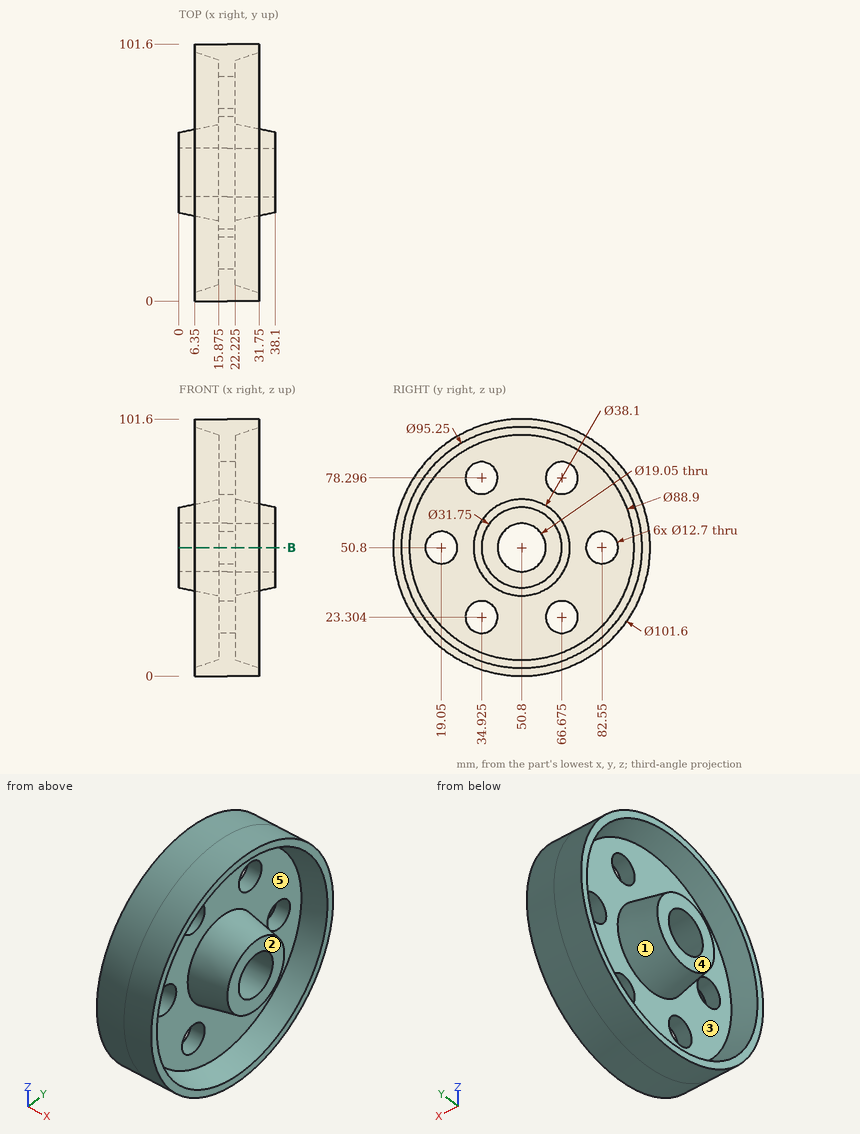
Answer from the drawing. Dimensions are ordinates in mm from the lowest x, y and z of the part. A direction names the side the tool comes from. Give positions to 0.01 mm unless a question says otherwise; leave off trailing zeros.
Item 1: Each of these flat-tipped pins is pushed along its axis until it touches: pin 1 Ø20.5 at (y, z) = (66.68, 23.3) entering from +X (3 decimals); pin 2 Ø1 at (x, z) = (22, 65) entering from -Y; pin 3 Ø8 at (x, z) = (16.5, 46.5) entering from +Y. Where does it stop, or does it pass through?
Item 2: Find the intervals of material crossed by line 1 along Y through (x, z) = (20.75, 50.8) (1 decimal); line 2 along Z through (x, y) = (26.5, 64.5) (1 decimal); line 3 along Z through (x, y) = (18.5, 64) (1 decimal), in increasing order.
Item 3: The part is cut by section B-B (z = 50.8). Give the number of separate pieces and of enclosed holes in the cut face, and give its area (3 significant figures).
Item 4: For the marked faces 3, 4 and 5, determine the directions among +Z, -Z, +X, -X, +Y, -Y from which every point of the face is accessible in a straight line to the end or side of a thin tool.
Item 5: The mould has two halves that part along Y. Classify the marked faces 1 and 2: released by +Y, released by -Y, zero draft, split by the parting line, or undercut.
Taken from the geometry:
1. pin 1: stops at x = 22.225
1. pin 2: stops at y = 1.88
1. pin 3: stops at y = 101.6
2. line 1: y = 0 to 12.7, 25.4 to 41.3, 60.3 to 76.2, 88.9 to 101.6
2. line 2: z = 1.9 to 7, 38.8 to 62.8, 94.6 to 99.7
2. line 3: z = 1.7 to 17.5, 29.1 to 72.5, 84.1 to 99.9
3. separate pieces: 4
3. enclosed holes: 0
3. area: 1,050 mm2
4. face 3: -X
4. face 4: +Z, -Z, -X, +Y, -Y
4. face 5: +X
5. face 1: undercut
5. face 2: zero draft
